from build123d import *

# Parameters (mm, degrees)
EXTRUDE_1_DEPTH     = 6
SKETCH_2_R          = 6
EXTRUDE_2_DEPTH     = 24
SKETCH_3_R          = 2.5
CUT_EXTRUDE_1_DEPTH = 24
SKETCH_4_R          = 2
CUT_EXTRUDE_2_DEPTH = 6


with BuildPart() as part:
    # 草图1 → 凸台-拉伸1 (new body)
    with BuildSketch(Plane(origin=(0, 0, 0), x_dir=(1, 0, 0), z_dir=(0, 1, 0))):
        Polygon((5.88746988, -3.652081381), (6.106530193, 3.27265779), (0.219060313, 6.92473917), (-5.88746988, 3.652081381), (-6.106530193, -3.27265779), (-0.219060313, -6.92473917), align=None)
    extrude(amount=EXTRUDE_1_DEPTH)

    # 草图2 → 凸台-拉伸2 (add)
    with BuildSketch(Plane(origin=(0, 6, 0), x_dir=(1, 0, 0), z_dir=(0, 1, 0))):
        with Locations(Location((0, 0, 0), (0, 0, 118.188083805))):
            Circle(SKETCH_2_R)
    extrude(amount=EXTRUDE_2_DEPTH)

    # 草图3 → 切除-拉伸1 (cut)
    with BuildSketch(Plane(origin=(0, 30, 0), x_dir=(1, 0, 0), z_dir=(0, 1, 0))):
        with Locations(Location((0, 0, 0), (0, 0, 270))):
            Circle(SKETCH_3_R)
    extrude(amount=-CUT_EXTRUDE_1_DEPTH, mode=Mode.SUBTRACT)

    # 草图4 → 切除-拉伸2 (cut)
    with BuildSketch(Plane.XZ):
        with Locations(Location((0, 0, 0), (0, 0, 270))):
            Circle(SKETCH_4_R)
    extrude(amount=-CUT_EXTRUDE_2_DEPTH, mode=Mode.SUBTRACT)


solid = part.part
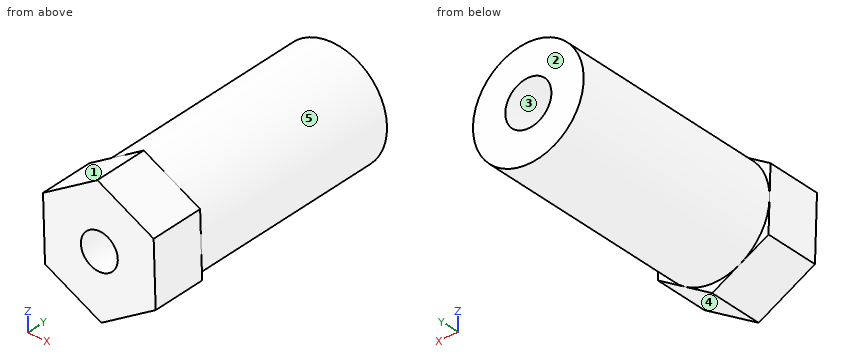
Can you work these out from the model? Positions are in its coordinate system, mm. Face numbers are marked on the shaded views. A direction names the side the tool comes from. Give positions to 0.01 mm unless a question says otherwise; leave off trailing zeros. Loops run counter-clockwise (first coordinate to the right, second up) from the corner with the lowest first, then second, coordinate; pieces in that order, holes last. Notation, with made-up numbers: (17, 62) - (22, 62) arc R20 cw to (22, 82) - close; hole circle Ø4 at (49.5, 62). An arc over 180 degrees is marked (long way). Answer as a JSON object with one key per item and string values.
Q1. Imagine slicing it at C-C on x = -3.75. Write out the boundary of the cut face in (y, z), plus the area to 3 significant figures.
Geometry says:
{"outline": "(0, -4.8) - (6, -4.8) - (6, -4.68) - (30, -4.68) - (30, 4.68) - (6, 4.68) - (6, 4.73) - (0, 4.73) - close", "area": "282 mm²"}
Q2. Imagine slicing it at B-B on z = -1. Write out the boundary of the cut face in (x, y), plus the area to 3 significant figures.
Geometry says:
{"outline": "(-5.97, 0) - (-1.73, 0) - (-1.73, 6) - (-2.29, 6) - (-2.29, 30) - (-5.92, 30) - (-5.92, 6) - (-5.97, 6) - close; (1.73, 0) - (6.03, 0) - (6.03, 6) - (5.92, 6) - (5.92, 30) - (2.29, 30) - (2.29, 6) - (1.73, 6) - close", "area": "225 mm²"}
Q3. If I drill on L1, parallel to X at y = 11.75, z = 0; L2, parallel to X at y = 2.55, z = 0; L3, parallel to Z at x = 1.75, y = 11.75, over which ranges is the centre line in solid material (lowest first)?
Geometry says:
{"L1": "-6 to -2.5, 2.5 to 6", "L2": "-6 to -2, 2 to 6", "L3": "-5.74 to -1.79, 1.79 to 5.74"}
Q4. Which directions (+Z, -Z, +X, -X, +Y, -Y) give clear straight access to the entire face, cutting with the end or side of a thin tool? Please do the marked faces 4 and 5.
Geometry says:
{"face 4": "-Z, +X, +Y, -Y", "face 5": "+Y"}
Q5. Imagine slicing it at A-A on y = 12.5. Write out the boundary of the cut face in (x, z), plus the area to 3 significant figures.
Geometry says:
{"outline": "circle Ø12 at (0, 0); hole circle Ø5 at (0, 0)", "area": "93.5 mm²"}
Q6. Will this pin go through, and if not, where does the flat tip stop? P1, Ø5, axis at x = -1.5, y = 14.5, coming from the +Z side.
Geometry says:
{"P1": "z = 6"}
Q7. If we mould it in two halves opening along Z, with no side actions, what happens to the marked faces 1, 2 and 3? For each: pulls with the +Z half, pulls with the -Z half, needs draft (parallel to the pull), parting line crosses it, or undercut.
Geometry says:
{"face 1": "pulls with the +Z half", "face 2": "needs draft", "face 3": "undercut"}
